Geometry check sheet. Reference: drawing and pictorial views, mm from the part's lowest x, y, z. A direction names the side the tool comes from. Round coordinates to 2 decimals unless told otherwise and drop trailing zeros. Write each loop counter-clockwise with the first axis right and the second up, starting at its lowest first coordinate (ties: lowest second). Pieces come first, ordered by that corner, then holes. Notation, with made-up numbers: M -6.75,50 L 7.25,50 A14 ccw 7.25,76 Z; hole C 2.25,80.25 d7. An arc over 180 degrees is marked long. One line per question, with ' | ' between items.
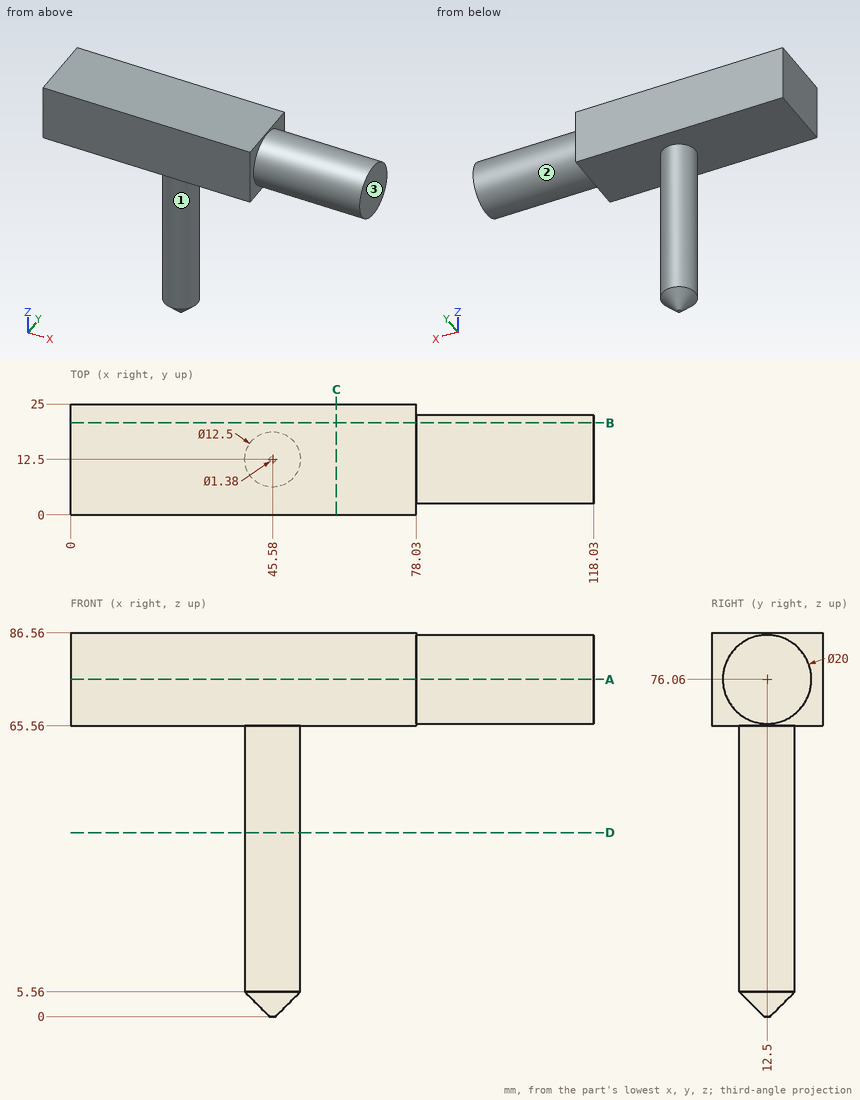
1. Section check A-A, the plane z = 76.06. Record the cut outline in (x, y).
Results:
outline: M 0,0 L 78.03,0 L 78.03,2.5 L 118.03,2.5 L 118.03,22.5 L 78.03,22.5 L 78.03,25 L 0,25 Z
2. Section check D-D, the plane z = 41.5. Record the cut outline in (x, y).
Results:
outline: C 45.58,12.5 d12.5
3. Section check B-B, the plane y = 20.75. Record the cut outline in (x, z), then the cut area to 3 significant figures.
Results:
outline: M 0,65.56 L 78.03,65.56 L 78.03,70.41 L 118.03,70.41 L 118.03,81.71 L 78.03,81.71 L 78.03,86.56 L 0,86.56 Z | area: 2,090 mm2
4. Tool access check on the marked faces 1, 2 and 3. Record the directions out of +Z, -Z, +X, -X, +Y, -Y that give a thin tool (end or side, any length) a straight path to the whole face; none if there is none.
Results:
face 1: -Z | face 2: +X | face 3: +Z, -Z, +X, +Y, -Y
5. Thickness scan on line 1 (Z direction, x = 17, y = 15.5); line 2 (X direction, y = 23.5, z = 79); line 3 (Y direction, x = 41, z = 14.5). Record the ranges inside material, lowest first.
Results:
line 1: z = 65.56 to 86.56 | line 2: x = 0 to 78.03 | line 3: y = 8.25 to 16.75
6. Section check C-C, the plane x = 60. Record the cut outline in (y, z).
Results:
outline: M 0,65.56 L 25,65.56 L 25,86.56 L 0,86.56 Z
7. Go/stop test with flat-tipped pins: P1, Ø6, axis at x = 82.5, y = 11, coming from the -Z side; P2, Ø6, axis at x = 94.5, y = 17.5, coming from the -Z side; P3, Ø5, axis at y = 4.5, z = 21.5, coming from the +X side. Record where each tip stops, or that it passes through.
Results:
P1: stops at z = 66.06 | P2: stops at z = 66.26 | P3: stops at x = 48.55
